```python
from build123d import *

# Parameters (mm, degrees)
SKETCH3_R           = 8.05
BOSS_EXTRUDE1_DEPTH = 8
SKETCH4_R           = 8.05
SKETCH4_R_2         = 4.3
BOSS_EXTRUDE2_DEPTH = 3
CHAMFER1_SIZE       = 3
FILLET1_R           = 11
SKETCH5_R           = 1.65
CUT_EXTRUDE1_DEPTH  = 85.020655349
SKETCH6_R           = 3
CUT_EXTRUDE2_DEPTH  = 3
SKETCH7_W           = 22
SKETCH7_H           = 25.1
CUT_EXTRUDE3_DEPTH  = 93.528214752
FILLET2_R           = 2
SKETCH8_R           = 1.65
CUT_EXTRUDE4_DEPTH  = 72.905914397
CUT_EXTRUDE5_DEPTH  = 72.905914397
FILLET3_R           = 5
SKETCH10_R          = 3
CUT_EXTRUDE6_DEPTH  = 3


with BuildPart() as part:
    # Sketch3 → Boss-Extrude1 (new body)
    with BuildSketch(Plane.XY):
        with BuildLine():
            Line((-31.937438845, -2), (-45.623026261, -2))
            Line((-45.623026261, -2), (-45.623026261, -10))
            Line((-45.623026261, -10), (-35.623026261, -10))
            ThreePointArc((-35.623026261, -10), (-26.529067588, -25.791637654), (-11, -35.327043465))
            Line((-11, -35.327043465), (-11, -80.1))
            Line((-11, -80.1), (11, -80.1))
            Line((11, -80.1), (11, -35.327043465))
            ThreePointArc((11, -35.327043465), (26.529067588, -25.791637654), (35.623026261, -10))
            Line((35.623026261, -10), (45.623026261, -10))
            Line((45.623026261, -10), (45.623026261, -2))
            Line((45.623026261, -2), (31.937438845, -2))
            ThreePointArc((31.937438845, -2), (0, -32), (-31.937438845, -2))
        make_face()
        with Locations((0, -69.1)):
            Circle(SKETCH3_R, mode=Mode.SUBTRACT)
    extrude(amount=BOSS_EXTRUDE1_DEPTH)

    # Sketch4 → Boss-Extrude2 (add)
    with BuildSketch(Plane.XY):
        with Locations(Location((0, -69.1, 0), (0, 0, 180))):
            Circle(SKETCH4_R)
        with Locations(Location((0, -69.1, 0), (0, 0, 180))):
            Circle(SKETCH4_R_2, mode=Mode.SUBTRACT)
    extrude(amount=BOSS_EXTRUDE2_DEPTH)

    # Chamfer1
    chamfer1_edges = [part.edges().sort_by_distance(p)[0] for p in [
        (0, -80.1, 0),
    ]]
    chamfer(chamfer1_edges, length=CHAMFER1_SIZE)

    # Fillet1
    fillet1_edges = [part.edges().sort_by_distance(p)[0] for p in [
        (-11, -80.1, 5.5),
        (11, -80.1, 5.5),
    ]]
    fillet(fillet1_edges, radius=FILLET1_R - 0.0001)  # a hair under: the kernel refuses the full size

    # Sketch5 → Cut-Extrude1 (cut, through all)
    with BuildSketch(Plane.XZ.offset(10)):
        with Locations((40.623026261, 4)):
            Circle(SKETCH5_R)
    cut_extrude1 = extrude(amount=-CUT_EXTRUDE1_DEPTH, mode=Mode.SUBTRACT)

    # Sketch6 → Cut-Extrude2 (cut)
    with BuildSketch(Plane.XZ.offset(10)):
        with Locations((40.623026261, 4)):
            Circle(SKETCH6_R)
    cut_extrude2 = extrude(amount=-CUT_EXTRUDE2_DEPTH, mode=Mode.SUBTRACT)

    # Mirror1: Cut-Extrude1, Cut-Extrude2 across plane
    add(cut_extrude1.mirror(Plane(origin=(0, 0, 0), x_dir=(0, 0, 1), z_dir=(1, 0, 0))), mode=Mode.SUBTRACT)
    add(cut_extrude2.mirror(Plane(origin=(0, 0, 0), x_dir=(0, 0, 1), z_dir=(1, 0, 0))), mode=Mode.SUBTRACT)

    # Sketch7 → Cut-Extrude3 (cut, through all)
    with BuildSketch(Plane.XY.offset(8)):
        with Locations((0, -67.55)):
            Rectangle(SKETCH7_W, SKETCH7_H)
    extrude(amount=-CUT_EXTRUDE3_DEPTH, mode=Mode.SUBTRACT)

    # Fillet2
    fillet2_edges = [part.edges().sort_by_distance(p)[0] for p in [
        (-45.623026261, -2, 4),
        (-31.937438845, -2, 4),
        (31.937438845, -2, 4),
        (45.623026261, -2, 4),
        (45.623026261, -10, 4),
        (35.623026261, -10, 4),
        (-35.623026261, -10, 4),
        (-45.623026261, -10, 4),
    ]]
    fillet(fillet2_edges, radius=FILLET2_R - 0.0001)  # a hair under: the kernel refuses the full size

    # Sketch8 → Cut-Extrude4 (cut, through all)
    with BuildSketch(Plane.XY.offset(8)):
        with Locations((4.5, -49)):
            Circle(SKETCH8_R)
        with Locations((-4.5, -49)):
            Circle(SKETCH8_R)
    extrude(amount=-CUT_EXTRUDE4_DEPTH, mode=Mode.SUBTRACT)

    # Sketch9 → Cut-Extrude5 (cut, through all)
    with BuildSketch(Plane.XY.offset(8)):
        with BuildLine():
            Line((-8.75, -55), (-8.75, -35.950486784))
            ThreePointArc((-8.75, -35.950486784), (-9.879918795, -35.656517001), (-11, -35.327043465))
            Line((-11, -35.327043465), (-11, -55))
            Line((-11, -55), (-8.75, -55))
        make_face()
        with BuildLine():
            Line((8.75, -55), (8.75, -35.950486784))
            ThreePointArc((8.75, -35.950486784), (9.879918795, -35.656517001), (11, -35.327043465))
            Line((11, -35.327043465), (11, -55))
            Line((11, -55), (8.75, -55))
        make_face()
    extrude(amount=-CUT_EXTRUDE5_DEPTH, mode=Mode.SUBTRACT)

    # Fillet3
    fillet3_edges = [part.edges().sort_by_distance(p)[0] for p in [
        (-8.75, -55, 4),
        (-8.75, -35.950486784, 4),
        (8.75, -55, 4),
        (8.75, -35.950486784, 4),
    ]]
    fillet(fillet3_edges, radius=FILLET3_R)

    # Sketch10 → Cut-Extrude6 (cut)
    with BuildSketch(Plane.XY.offset(8)):
        with Locations((4.5, -49)):
            Circle(SKETCH10_R)
        with Locations((-4.5, -49)):
            Circle(SKETCH10_R)
    extrude(amount=-CUT_EXTRUDE6_DEPTH, mode=Mode.SUBTRACT)


solid = part.part
```
Verification items for the finished model (mm, model axes). A direction names the side the tool comes from. Round coordinates to 2 decimals unless told otherwise and drop trailing zeros. Write each loop counter-clockwise with the first axis right and the second up, starting at its lowest first coordinate (ties: lowest second). Pieces come first, ordered by that corner, then holes. Notation, with made-up numbers: (49, 76) - (97, 76) arc R24 ccw to (97, 113) - close; hole circle Ø2 at (45, 3.5). An arc over 180 degrees is marked (long way). Answer as a JSON object with one key per item and string values. Group by question number.
Q1. Mould release check, pull along X, two halves, no side actions. Record for faces 6 (the cylindrical face through (-45.05, -2.6, 4.06)), 7 (the flat face through (0, -55, 4)), 8 (the flat face through (-41.9, -7, 2.7)): released by +X, released by -X, zero draft, split by the parting line, or undercut.
Q2. Tool access check on faces 1 (the flat face through (8.75, -45, 4)), 2 (the flat face through (-38.6, -2, 3.9)), 3 (the flat face through (-3, -50, 5)), 4 (the cylindrical face through (43.484, -8.521, 4.901)), 5 (the flat face through (-8.75, -45, 4)). Record the directions out of +Z, -Z, +X, -X, +Y, -Y that give a thin tool (end or side, any length) a straight path to the whole face; none if there is none.
Q3. Section check B-B, the plane z = 4. Give the number of separate pieces and of enclosed holes in the cut face, plus the area to 3 significant figures.
Q4. Go/stop test with flat-tipped pins: pin 1 Ø3.5 at (x, z) = (39, 5) entering from -Y; pin 2 Ø3 at (x, z) = (-40, 3.5) entering from -Y; pin 3 Ø4 at (y, z) = (-43.5, 3) entering from +X. Record where each tip stops, or that it passes through.
Q5. Thickness scan on line 1 (X direction, y = -5, z = 5.25); line 2 (X direction, y = -16.5, z = 3); line 3 (X direction, y = -14, z = 5.5). Record the ranges inside material, lowest first.
Q6. Section check A-A, the plane y = -49. Enter the section's corners in (x, z).
Found:
{
 "1": {"face 6": "released by -X", "face 7": "zero draft", "face 8": "undercut"},
 "2": {"face 1": "+Z, -Z, +X, -Y", "face 2": "+Z, -Z, +X, -X, +Y", "face 3": "+Z", "face 4": "-Y", "face 5": "+Z, -Z, -X, -Y"},
 "3": {"separate pieces": "3", "enclosed holes": "2", "area": "894 mm^2"},
 "4": {"pin 1": "stops at y = -10", "pin 2": "stops at y = -7", "pin 3": "stops at x = 8.75"},
 "5": {"line 1": "x = -45.62 to -41.7, -39.55 to -31.61, 31.61 to 39.55, 41.7 to 45.62", "line 2": "x = -33.12 to -27.42, 27.42 to 33.12", "line 3": "x = -34.25 to -28.77, 28.77 to 34.25"},
 "6": {"outline": "(-8.75, 0) - (-6.15, 0) - (-6.15, 5) - (-7.5, 5) - (-7.5, 8) - (-8.75, 8) - close; (-2.85, 0) - (2.85, 0) - (2.85, 5) - (1.5, 5) - (1.5, 8) - (-1.5, 8) - (-1.5, 5) - (-2.85, 5) - close; (6.15, 0) - (8.75, 0) - (8.75, 8) - (7.5, 8) - (7.5, 5) - (6.15, 5) - close"}
}
